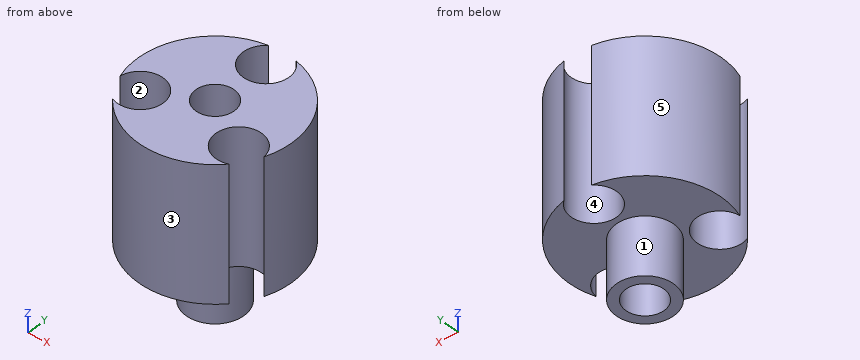
```python
from build123d import *

# Parameters (mm, degrees)
F0_R     = 25.4
F1_DEPTH = 44.45
F2_R     = 9.525
F3_DEPTH = 19.05
F4_R     = 6.35
F5_DEPTH = 76.2
F6_R     = 7.581193
F7_DEPTH = 44.45


with BuildPart() as f1:
    # F0 (on Top) → F1 (new body)
    with BuildSketch(Plane.XY):
        Circle(F0_R)
    extrude(amount=F1_DEPTH)

    # F2 (on Top) → F3 (join)
    with BuildSketch(Plane.XY):
        Circle(F2_R)
    extrude(amount=-F3_DEPTH)

    # F4 (on face) → F5 (cut)
    with BuildSketch(Plane(origin=(0, 0, -19.05), x_dir=(1, 0, 0), z_dir=(0, 0, -1))):
        Circle(F4_R)
    extrude(amount=-F5_DEPTH, mode=Mode.SUBTRACT)

    # F6 (on Top) → F7 (cut)
    with BuildSketch(Plane.XY):
        with Locations((0, 18.949738)):
            Circle(F6_R)
        with Locations((-16.410954, -9.474869)):
            Circle(F6_R)
        with Locations((16.410954, -9.474869)):
            Circle(F6_R)
    extrude(amount=F7_DEPTH, mode=Mode.SUBTRACT)


solid = f1.part
```
Here's how the part is built. I have some questions about the finished solid (model axes, mm). Face numbers are marked on the shaded views. A direction names the side the tool comes from. Give positions to 0.01 mm unless a question says otherwise; leave off trailing zeros. Loops run counter-clockwise (first coordinate to the right, second up) from the corner with the lowest first, then second, coordinate; pieces in that order, holes last. Notation, with made-up numbers: M 50,18 L 58,18 A28 cw 58,37 Z; hole C 22,-19.75 d3. An arc over 180 degrees is marked long. Put each result on its own line as item: value. Start each with the question number.
(1) I want a section at A-A on x = 0. Please give me the cut outline in (y, z) (3 decimals), then the cut area to 3 significant figures.
(2) I want a section at D-D on y = 16.5. Please give me the cut outline in (x, z), then the cut area to 3 significant figures.
(3) For the marked faces 1 and 2, which set-ups out of +Z, -Z, +X, -X, +Y, -Y let a thin tool reach every point of the face, with its end or its side?
(4) If we mould it in two halves opening along X, with no side actions, what happens to the marked faces 3, 4 and 5? For each: +X half, -X half, draft (parallel to the pull), parting line (faces both ways), or undercut.
(5) Will these pins go through, and if not, where does the flat tip stop? pin 1 Ø3 at (x, z) = (-2, 10.5) entering from -Y; pin 2 Ø3 at (x, y) = (-10.5, -11.5) entering from -Z; pin 3 Ø5 at (y, z) = (10.5, 7.5) entering from -X; pin 4 Ø1.5 at (x, z) = (-17.5, -2) entering from +Y.
(6) I want a section at B-B on y = 0. Please give me the cut outline in (x, z) (3 decimals), then the cut area to 3 significant figures.
(7) I need wall thicknesses on line 1 along X through (y, z) = (0, 24); line 2 along Z through (x, y) = (8.5, -8); line 3 along Y through (x, z) = (-3, 36.5). Which ranges of each line are inside material? Lowest first, please. Write a range as [from, to].
(8) I want a section at C-C on z = 38. Please give me the cut outline in (x, y).
Answer block:
1. outline: M -25.4,0 L -9.525,0 L -9.525,-19.05 L -6.35,-19.05 L -6.35,44.45 L -25.4,44.45 Z; M 6.35,-19.05 L 9.525,-19.05 L 9.525,0 L 11.369,0 L 11.369,44.45 L 6.35,44.45 Z
1. area: 1,190 mm^2
2. outline: M -19.31,0 L -7.17,0 L -7.17,44.45 L -19.31,44.45 Z; M 7.17,0 L 19.31,0 L 19.31,44.45 L 7.17,44.45 Z
2. area: 1,080 mm^2
3. face 1: -Z
3. face 2: +Z, -Z
4. face 3: parting line
4. face 4: undercut
4. face 5: -X half
5. pin 1: y = -25.4
5. pin 2: z = 0
5. pin 3: x = -24.11
5. pin 4: through
6. outline: M -25.4,0 L -9.525,0 L -9.525,-19.05 L -6.35,-19.05 L -6.35,44.45 L -25.4,44.45 Z; M 6.35,-19.05 L 9.525,-19.05 L 9.525,0 L 25.4,0 L 25.4,44.45 L 6.35,44.45 Z
6. area: 1,810 mm^2
7. line 1: [-25.4, -6.35], [6.35, 25.4]
7. line 2: [0, 44.45]
7. line 3: [-25.22, -5.6], [5.6, 11.99]
8. outline: M -23.93,-8.51 A7.58 cw long -19.34,-16.47 A25.4 ccw 19.34,-16.47 A7.58 cw long 23.93,-8.51 A25.4 ccw 4.59,24.98 A7.58 cw long -4.59,24.98 A25.4 ccw Z; hole C 0,0 d12.7
